Geometry: final body of the model. Coordinates: model frame, mm. Face numbers are marked on the shaded views. Coordinates: 2 decimals unless noted, no trailing zeros. Write each loop counter-clockwise with the first axis right and the second up, starting at its lowest first coordinate (ties: lowest second). Pieces come first, ordered by that corner, then holes. Notation, with made-up numbers: (15, -29.5) - (53, -29.5) arc R25 ccw to (53, -13.5) - close; hole circle Ø8 at (50, -2.75). An arc over 180 degrees is marked (long way). Answer as a JSON object with one key per item and string values. Group by question number.
Item 1: Line query: line 1 along Y through (x, z) = (74, -1.25); line 2 along Y through (x, z) = (45, -7.5); line 3 along Y through (x, z) = (127.5, -1.25). Output: solid intervals per line, ascending. Write a range as from..to.
Item 2: Mould query, pull axis X, two halves, no side actions, for the marked faces 1 and 2. Classes: pulls with the +X half, pulls with the -X half, needs draft (parallel to the pull), parting line crosses it, or undercut.
Item 3: First-contact query: pin 1 Ø3 at (y, z) = (60, -6.5) entering from -X; pin 2 Ø3 at (y, z) = (61, -4.5) entering from +X; pin 3 Ø2.5 at (x, z) = (67.5, -2) entering from -Y. Flat tips, straight axial feed; report the tip coordinate or a pass-through.
Item 4: Section C-C on x = 33.5. Return loops of the section in (y, z).
Item 5: Section B-B on x = 98. Return loops of the section in (y, z).
Item 6: Section D-D on y = 38.5. Return loops of the section in (x, z), and give its area (3 significant figures).
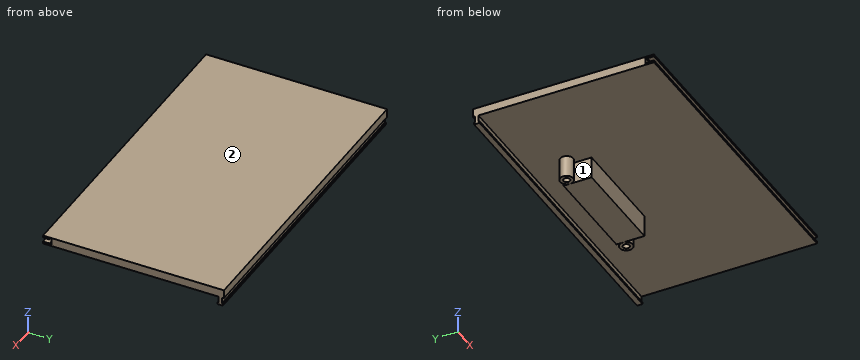
```python
from build123d import *

# Parameters (mm, degrees)
SKETCH185_W     = 145
SKETCH185_H     = 84
PAD088_DEPTH    = 4
SKETCH186_W     = 1.5
SKETCH186_H     = 3
SKETCH186_W_2   = 2.5
SKETCH186_H_2   = 0.9
PAD089_DEPTH    = 145
SKETCH187_W     = 3
SKETCH187_H     = 2
SKETCH187_W_2   = 1
SKETCH187_H_2   = 3
POCKET109_DEPTH = 145
SKETCH188_R     = 3
SKETCH188_W     = 47
SKETCH188_H     = 13
PAD090_DEPTH    = 10
SKETCH189_R     = 1.5
POCKET110_DEPTH = 7


with BuildPart() as part:
    # Sketch185 → Pad088 (new body)
    with BuildSketch(Plane.XY):
        with Locations((72.5, 42)):
            Rectangle(SKETCH185_W, SKETCH185_H)
    extrude(amount=PAD088_DEPTH)

    # Sketch186 → Pad089 (join)
    with BuildSketch(Plane.YZ):
        with Locations((82.25, -1.5)):
            Rectangle(SKETCH186_W, SKETCH186_H)
        with Locations((82.25, -3.45)):
            Rectangle(SKETCH186_W_2, SKETCH186_H_2)
    extrude(amount=PAD089_DEPTH)

    # Sketch187 → Pocket109 (cut)
    with BuildSketch(Plane.YZ):
        with Locations((1.5, 2)):
            Rectangle(SKETCH187_W, SKETCH187_H)
        with Locations((3.5, 2)):
            Rectangle(SKETCH187_W_2, SKETCH187_H_2)
    extrude(amount=POCKET109_DEPTH, mode=Mode.SUBTRACT)

    # Sketch188 → Pad090 (join)
    with BuildSketch(Plane.XY):
        with Locations((98, 64)):
            Circle(SKETCH188_R)
        with Locations((45, 64)):
            Circle(SKETCH188_R)
        with Locations((71.5, 60.5)):
            Rectangle(SKETCH188_W, SKETCH188_H)
    extrude(amount=-PAD090_DEPTH)

    # Sketch189 (on Face1 of Pad090) → Pocket110 (cut)
    with BuildSketch(Plane(origin=(0, 0, -10), x_dir=(1, 0, 0), z_dir=(0, 0, -1))):
        with Locations((45, -64)):
            Circle(SKETCH189_R)
        with Locations((98, -64)):
            Circle(SKETCH189_R)
    extrude(amount=-POCKET110_DEPTH, mode=Mode.SUBTRACT)


solid = part.part
```
Checks:
{
 "1": {"line 1": "54..67, 81.5..83", "line 2": "61..62.5, 65.5..67", "line 3": "81.5..83"},
 "2": {"face 1": "undercut", "face 2": "needs draft"},
 "3": {"pin 1": "x = 43.34", "pin 2": "x = 100.6", "pin 3": "y = 54"},
 "4": {"outline": "(0, 0) - (81.5, 0) - (81.5, -3) - (81, -3) - (81, -3.9) - (83.5, -3.9) - (83.5, -3) - (83, -3) - (83, 0) - (84, 0) - (84, 4) - (0, 4) - (0, 3) - (3, 3) - (3, 3.5) - (4, 3.5) - (4, 0.5) - (3, 0.5) - (3, 1) - (0, 1) - close"},
 "5": {"outline": "(0, 0) - (61, 0) - (61, -10) - (62.5, -10) - (62.5, -3) - (65.5, -3) - (65.5, -10) - (67, -10) - (67, 0) - (81.5, 0) - (81.5, -3) - (81, -3) - (81, -3.9) - (83.5, -3.9) - (83.5, -3) - (83, -3) - (83, 0) - (84, 0) - (84, 4) - (0, 4) - (0, 3) - (3, 3) - (3, 3.5) - (4, 3.5) - (4, 0.5) - (3, 0.5) - (3, 1) - (0, 1) - close"},
 "6": {"outline": "(0, 0) - (145, 0) - (145, 4) - (0, 4) - close", "area": "580 mm^2"}
}
